```python
from build123d import *

# Parameters (mm, degrees)
ESBO_O2_R             = 28.575
CORTE_EXTRUS_O1_DEPTH = 10.7188


with BuildPart() as part:
    # Esboço1 → Revolução1 (revolve)
    with BuildSketch(Plane.XY):
        Polygon((0, 0), (0, 14.5923), (3.175, 17.7673), (7.5438, 17.7673), (10.7188, 14.5923), (10.7188, 0), align=None)
    revolve(axis=Axis((10.7188, 0, 0), (-1, 0, 0)))

    # Esboço2 → Corte-extrusão1 (cut)
    with BuildSketch(Plane(origin=(0, 0, 0), x_dir=(0, 0, -1), z_dir=(1, 0, 0))):
        Circle(ESBO_O2_R)
        Polygon((-14.2875, -8.248891971), (0, -16.497783942), (14.2875, -8.248891971), (14.2875, 8.248891971), (0, 16.497783942), (-14.2875, 8.248891971), align=None, mode=Mode.SUBTRACT)
    extrude(amount=CORTE_EXTRUS_O1_DEPTH, mode=Mode.SUBTRACT)

    # Esboço3 → Corte-Revolução1 (revolve, cut)
    with BuildSketch(Plane.XY):
        Polygon((0, 0), (0, 9.525), (0.68707, 8.83793), (10.03173, 8.83793), (10.7188, 9.525), (10.7188, 0), align=None)
    revolve(axis=Axis((10.7188, 0, 0), (-1, 0, 0)), mode=Mode.SUBTRACT)


solid = part.part
```
Could you check a few things on this model? Use its own coordinates, in mm. Coordinates: 2 decimals unless noted, no trailing zeros. Order: outer loops, then holes, each group sorted by start corner. A loop starts at its lowest first (then second) coordinate and runs counter-clockwise, first axis right, second up. Notation, with made-up numbers: M -7.75,-7.75 L 33.25,-7.75 A22 cw 33.25,30.25 Z; hole C 74,54 d4. An arc over 180 degrees is marked long. Use one line per item in the form item = value. Start each with the question number.
1. For pin 1 (4 mm diameter, centred on x = 8, z = -11.5, fed in from +Y); pin 2 (5 mm diameter, centred on x = 5, y = -11.5, fed in from -Z); pin 3 (2 mm diameter, centred on x = 4, y = 12.5, fed in from -Z), each with a flat end and sliding along its axis, tell me the tip position at first contact or that it passes through.
2. Suppose I cut it at B-B on x = 1.5. Write out the boundary of the cut face in (y, z), then the cut area to 3 significant figures.
3. We'd pull the mould along Z, two halves only. Please class faces 1 (the cylindrical face through (5.425, -1.151, -8.763)), 2 (the conical face through (10.2, -7.5, -13.12)), 3 (the conical face through (10.2, 7.5, 13.12)), 4 (the conical face through (10.2, -15.11, -0.07)): +Z half, -Z half, draft (parallel to the pull), parting line (faces both ways), or undercut.
4. Suppose I cut it at A-A on y = 0. Write out the boundary of the cut face in (x, z) (1 decimal), then the cut area to 3 significant figures.
5. Please list where these lines run through material, in increasing order: line 1 (Y direction, x = 2.75, z = 0); line 2 (Z direction, x = 4, y = 0); line 3 (Y direction, x = 5.5, z = 3).
Geometry says:
q1.pin_1 = 11.01
q1.pin_2 = -12.99
q1.pin_3 = -8.66
q2.outline = M -16.08,-0.73 L -8.67,-13.56 A16.09 ccw -7.4,-14.29 L 7.4,-14.29 A16.09 ccw 8.67,-13.56 L 16.08,-0.73 A16.09 ccw 16.08,0.73 L 8.67,13.56 A16.09 ccw 7.4,14.29 L -7.4,14.29 A16.09 ccw -8.67,13.56 L -16.08,0.73 A16.09 ccw Z; hole C 0,0 d17.68
q2.area = 460 mm^2
q3.face_1 = undercut
q3.face_2 = -Z half
q3.face_3 = +Z half
q3.face_4 = parting line
q4.outline = M 0,-14.3 L 10.7,-14.3 L 10.7,-9.5 L 10,-8.8 L 0.7,-8.8 L 0,-9.5 Z; M 0,9.5 L 0.7,8.8 L 10,8.8 L 10.7,9.5 L 10.7,14.3 L 0,14.3 Z
q4.area = 116 mm^2
q5.line_1 = -16.5 to -8.84, 8.84 to 16.5
q5.line_2 = -14.29 to -8.84, 8.84 to 14.29
q5.line_3 = -14.77 to -8.31, 8.31 to 14.77
